from build123d import *

# Parameters (mm, degrees)
BOSS_EXTRUDE1_DEPTH = 20
CUT_EXTRUDE1_DEPTH  = 15
FILLET1_R           = 2
SKETCH3_R           = 1.5
CUT_EXTRUDE2_DEPTH  = 31.083311404
SKETCH4_R           = 1.5
CUT_EXTRUDE3_DEPTH  = 31.083311404
SCALE1_SCALE        = 1.02


with BuildPart() as part:
    # Sketch1 → Boss-Extrude1 (new body)
    with BuildSketch(Plane(origin=(0, 0, 0), x_dir=(0, 0, -1), z_dir=(1, 0, 0))):
        Polygon((0, -12.5), (-3.175, -12.5), (-6.175, -12.5), (-6.175, 6.175), (12.5, 6.175), (12.5, 3.175), (12.5, 0), (12.5, -3), (3, -12.5), align=None)
    extrude(amount=BOSS_EXTRUDE1_DEPTH)

    # Sketch2 → Cut-Extrude1 (cut)
    with BuildSketch(Plane(origin=(20, 0, 0), x_dir=(0, 0, -1), z_dir=(1, 0, 0))):
        Polygon((-3.175, -12.5), (0, -12.5), (0, 0), (12.5, 0), (12.5, 3.175), (-3.175, 3.175), align=None)
    extrude(amount=-CUT_EXTRUDE1_DEPTH, mode=Mode.SUBTRACT)

    # Fillet1
    fillet1_edges = [part.edges().sort_by_distance(p)[0] for p in [
        (20, -4.6625, 3.175),
        (20, -6.25, 0),
        (20, 0, -6.25),
        (20, 3.175, -4.6625),
    ]]
    fillet(fillet1_edges, radius=FILLET1_R)

    # Sketch3 → Cut-Extrude2 (cut, through all)
    with BuildSketch(Plane(origin=(0, 6.175, 0), x_dir=(1, 0, 0), z_dir=(0, 1, 0))):
        with Locations(Location((12.5, 6, 0), (0, 0, 90))):
            Circle(SKETCH3_R)
    extrude(amount=-CUT_EXTRUDE2_DEPTH, mode=Mode.SUBTRACT)

    # Sketch4 → Cut-Extrude3 (cut, through all)
    with BuildSketch(Plane.XY.offset(6.175)):
        with Locations((12.5, -6)):
            Circle(SKETCH4_R)
    extrude(amount=-CUT_EXTRUDE3_DEPTH, mode=Mode.SUBTRACT)


with BuildPart() as part_1:
    # Scale1: scaled about (9.068575954, -2.293993837, -2.293993837)
    add(part.part.scale(SCALE1_SCALE).moved(Location((-0.181371519, 0.045879877, 0.045879877))))


solid = part_1.part
Build history of the part. All positions in model axes, mm. A direction names the side the tool comes from. Give positions to 0.01 mm unless a question says otherwise; leave off trailing zeros. Order: outer loops, then holes, each group sorted by start corner. A loop starts at its lowest first (then second) coordinate and runs counter-clockwise, first axis right, second up. Notation, with made-up numbers: M 50.5,68 L 76.5,68 A29 ccw 76.5,91 Z; hole C 27.25,75.5 d6. An arc over 180 degrees is marked long. Use one line per item in the form item = value.
Q1. Slice it at C-C, the plane z = -7. Write the cut outline in (x, y).
Conclusion:
outline = M -0.18,-8.72 L 11.35,-8.72 L 11.35,-7 A1.53 cw 11.35,-5.15 L 11.35,0.05 L 4.92,0.05 L 4.92,3.28 L 11.35,3.28 L 11.35,6.34 L -0.18,6.34 Z; M 13.79,-8.72 L 20.22,-8.72 L 20.22,-1.99 A2.04 ccw 18.18,0.05 L 13.79,0.05 L 13.79,-5.15 A1.53 cw 13.79,-7 Z; M 13.79,3.28 L 18.18,3.28 A2.04 ccw 20.22,5.32 L 20.22,6.34 L 13.79,6.34 Z
Q2. Pin check, flat tips, straight feed: P1, Ø1.8, axis at x = 12.57, y = -6.07, coming from the -Z side; P2, Ø3.5, axis at x = 12.57, y = -6.07, coming from the -Z side; P3, Ø6, axis at x = 18, z = -9, coming from the -Y side. Stop position of each tip, or through.
Conclusion:
P1 = through
P2 = -11.4
P3 = -9.72
Q3. Pull direction Y, two halves, no side cores. Call faces 4 (the flat face through (12, 0.046, -8)), 5 (the cylindrical face through (11.28, 4.84, -6.9)), 6 (the flat face through (9.88, -7.79, -7.93)), 7 (the flat face through (10, 6.344, -3)): released by +Y, released by -Y, zero draft, split by the parting line, or undercut.
Conclusion:
face_4 = undercut
face_5 = zero draft
face_6 = released by -Y
face_7 = released by +Y
Q4. Slice it at A-A, the plane z = -2.5. Write the cut outline in (x, y), and give its area (3 significant figures).
Conclusion:
outline = M -0.18,-12.7 L 20.22,-12.7 L 20.22,-1.99 A2.04 ccw 18.18,0.05 L 4.92,0.05 L 4.92,3.28 L 18.18,3.28 A2.04 ccw 20.22,5.32 L 20.22,6.34 L -0.18,6.34 Z; hole C 12.57,-6.07 d3.06
area = 330 mm2
Q5. Wall check: probe 1 along Y at (x, z) = (15.75, -1); probe 2 along Z at (x, y) = (8, -9.75). Give the ranges that are in metal, low to high.
Conclusion:
probe_1 = -12.7 to 0.05, 3.28 to 6.34
probe_2 = -5.97 to 0.05, 3.28 to 6.34
Q6. Slice it at D-D, the plane y = 2.5. Write the cut outline in (x, z).
Conclusion:
outline = M -0.18,-12.7 L 4.92,-12.7 L 4.92,3.28 L 18.18,3.28 A2.04 ccw 20.22,5.32 L 20.22,6.34 L -0.18,6.34 Z
Q7. Slice it at B-B, the plane x = 5.25. Write the cut outline in (y, z), and give its area (3 significant figures).
Conclusion:
outline = M -12.7,-3.01 L -3.01,-12.7 L 0.05,-12.7 L 0.05,0.05 L -12.7,0.05 Z; M -12.7,3.28 L 3.28,3.28 L 3.28,-12.7 L 6.34,-12.7 L 6.34,6.34 L -12.7,6.34 Z
area = 223 mm2
Q8. Which spindle directions (+Z, -Z, +X, -X, +Y, -Y) get a long thin tool onto all of the face, cutting with end or side? Do faces 1 (the flat face through (9.9, -12.704, -0.3)), 2 (the flat face through (10, 3.284, -5)), 3 (the flat face through (12, -8, 0.046)). Say none if no direction does.
Conclusion:
face_1 = +Z, -Z, +X, -X, -Y
face_2 = -Z, +X
face_3 = +X, -Y
